from build123d import *

# Parameters (mm, degrees)
ESBO_O1_R                = 22
RESSALTO_EXTRUS_O1_DEPTH = 30
ESBO_O2_W                = 51.6
ESBO_O2_H                = 51.6
RESSALTO_EXTRUS_O2_DEPTH = 20
CORTE_EXTRUS_O4_REACH    = 52
ESBO_O17_W               = 51.6
ESBO_O17_H               = 51.6
ESBO_O17_R               = 25
ESBO_O18_R               = 2.5
CORTE_EXTRUS_O5_DEPTH    = 15


with BuildPart() as part:
    # Esboço1 → Ressalto-extrusão1 (new body)
    with BuildSketch(Plane(origin=(0, 0, 0), x_dir=(1, 0, 0), z_dir=(0, 1, 0))):
        Circle(ESBO_O1_R)
    extrude(amount=RESSALTO_EXTRUS_O1_DEPTH)

    # Esboço2 → Ressalto-extrusão2 (add)
    with BuildSketch(Plane.XZ):
        Rectangle(ESBO_O2_W, ESBO_O2_H)
    extrude(amount=RESSALTO_EXTRUS_O2_DEPTH)

    # Esboço13 → Broca de rosquear para tarraxa de M52 (revolve, cut)
    with BuildSketch(Plane(origin=(0, 15, 25.8), x_dir=(0, -1, 0), z_dir=(1, 0, 0))):
        Polygon((0, 0), (0, 16.2618073), (2.1, 15), (2.1, 0), align=None)
    broca_de_rosquear_para_tarraxa_de_m52 = revolve(axis=Axis((0, 15, 32.15), (0, 0, -1)), mode=Mode.SUBTRACT)

    # Espelhar1: Broca de rosquear para tarraxa de M52 across plane
    add(broca_de_rosquear_para_tarraxa_de_m52.mirror(Plane.XY), mode=Mode.SUBTRACT)

    # Esboço17 → Corte-extrusão4 (cut, up to next)
    with BuildSketch(Plane.XZ.offset(20), mode=Mode.PRIVATE) as corte_extrus_o4_sk1:
        Rectangle(ESBO_O17_W, ESBO_O17_H)
        Circle(ESBO_O17_R, mode=Mode.SUBTRACT)
    corte_extrus_o4_tool1 = extrude(corte_extrus_o4_sk1.sketch, amount=-CORTE_EXTRUS_O4_REACH, mode=Mode.PRIVATE) & part.part
    add(corte_extrus_o4_tool1.solids().sort_by_distance((25.070266, -20, 0))[0], mode=Mode.SUBTRACT)

    # Esboço18 → Corte-extrusão5 (cut)
    with BuildSketch(Plane.XZ.offset(20)):
        with Locations((8.838834765, 8.838834765)):
            Circle(ESBO_O18_R)
        with Locations((-8.838834765, 8.838834765)):
            Circle(ESBO_O18_R)
        with Locations((8.838834765, -8.838834765)):
            Circle(ESBO_O18_R)
        with Locations((-8.838834765, -8.838834765)):
            Circle(ESBO_O18_R)
    extrude(amount=-CORTE_EXTRUS_O5_DEPTH, mode=Mode.SUBTRACT)


solid = part.part
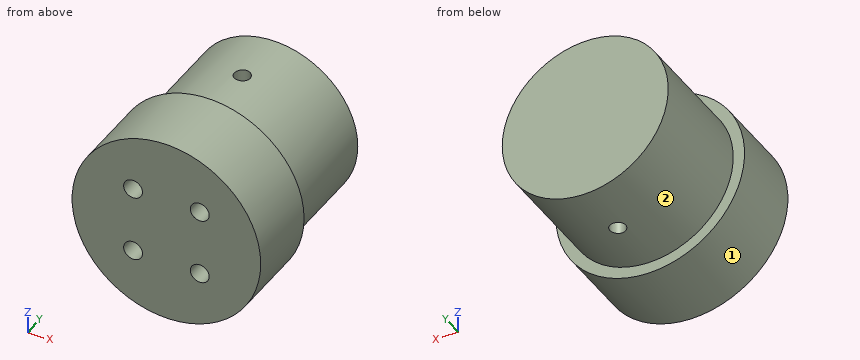
For this review, take the finished solid that the model builds, in its own axes (mm). Face numbers are marked on the shaded views. A direction names the side the tool comes from. Give positions to 0.01 mm unless a question says otherwise; leave off trailing zeros. Loops run counter-clockwise (first coordinate to the right, second up) from the corner with the lowest first, then second, coordinate; pieces in that order, holes last. Notation, with made-up numbers: M -17,-5.5 L 32,-5.5 A22 ccw 32,3.5 Z; hole C -25.5,-12.5 d4. An arc over 180 degrees is marked long. Answer as a JSON object with one key per item and string values. Group by question number.
Q1. Tool access review of the marked faces 1 and 2: name each direction out of +Z, -Z, +X, -X, +Y, -Y from which nothing blocks a thin tool from reaching the whole face with its end or side.
Q2. Add section C-C on x = -15.5. Give the boundary of the cut face in (y, z).
Q3. Add section B-B on y = -6. Give the boundary of the cut face in (x, z), and give its area (3 significant figures).
Q4. Add section A-A on z = 20. Give the boundary of the cut face in (x, y), and give its area (3 significant figures).
Q5. Add section D-D on z = 0. Give the boundary of the cut face in (x, y).
Q6. For probe 1 along Y at (x, z) = (0, -19); probe 2 along Z at (x, y) = (10.5, -14); probe 3 along Z at (x, y) = (0, -7), list the stretches that pass through material, from the lowest coordinate up. Write a range as [from, to].
Q7. Insertion check: P1, Ø8, axis at x = -16.5, y = 7.5, coming from the -Z side; P2, Ø10, axis at x = -17, y = -2.5, coming from the +Z side; P3, Ø1.5, axis at x = 8.5, z = 8, coming from the -Y side. Each pin has a flat end and moves straight along its axis. Give the tip position at first contact, or say it passes through.
Checked values:
{
 "1": {"face 1": "+Y, -Y", "face 2": "+Y"},
 "2": {"outline": "M -20,-19.62 L 0,-19.62 L 0,-15.61 L 30,-15.61 L 30,15.61 L 0,15.61 L 0,19.62 L -20,19.62 Z"},
 "3": {"outline": "C 0,0 d50; hole C -8.84,-8.84 d5; hole C -8.84,8.84 d5; hole C 8.84,-8.84 d5; hole C 8.84,8.84 d5", "area": "1,880 mm²"},
 "4": {"outline": "M -15,-20 L 15,-20 L 15,0 L 9.17,0 L 9.17,30 L -9.17,30 L -9.17,0 L -15,0 Z; hole C 0,15 d4.2", "area": "1,140 mm²"},
 "5": {"outline": "M -25,-20 L 25,-20 L 25,0 L 22,0 L 22,30 L -22,30 L -22,0 L -25,0 Z"},
 "6": {"probe 1": "[-20, 12.9], [17.1, 30]", "probe 2": "[-22.69, -10.71], [-6.97, 6.97], [10.71, 22.69]", "probe 3": "[-25, 25]"},
 "7": {"P1": "z = -18.1", "P2": "z = 21.93", "P3": "y = -5"}
}
